```python
from build123d import *

# Parameters (mm, degrees)
EXTRUDE_1_DEPTH = 30


with BuildPart() as part:
    # 草图1 → 凸台-拉伸1 (new body)
    with BuildSketch(Plane.XY):
        with BuildLine():
            Line((-89.550424061, 9.743331503), (-65.958441791, 33.335313773))
            Line((-65.958441791, 33.335313773), (14.763144604, -47.386272621))
            add(Edge.make_bspline(
                [(14.763144604, -47.386272621), (0.494407811, -57.892318184), (-24.857012127, -59.689840271), (-58.186688521, -56.851240275), (-88.692238529, -45.382338902), (-109.075510722, -32.199451169), (-119.928178624, -20.63442306)],
                knots=[0, 0, 0, 0, 0.341115549, 0.507979438, 0.680177262, 1, 1, 1, 1], degree=3))
            Line((-119.928178624, -20.63442306), (-140.199044416, -40.51331885))
            add(Edge.make_bspline(
                [(-140.199044416, -40.51331885), (-132.851023827, -52.488780749), (-122.952075778, -62.464006208)],
                knots=[0, 0, 0, 1, 1, 1], degree=2))
            Line((-122.952075778, -62.464006208), (-124.511456774, -64.591840844))
            ThreePointArc((-124.511456774, -64.591840844), (-142.61936624, -98.390264744), (-108.909761073, -80.117542921))
            Line((-108.909761073, -80.117542921), (-106.018688387, -77.202324863))
            add(Edge.make_bspline(
                [(-106.018688387, -77.202324863), (-93.714859758, -86.031565942), (-72.92911338, -97.233004689), (-42.077489767, -104.91243417), (-17.024761238, -104.223351741), (14.056661387, -100.072035401), (36.008728716, -91.143735824), (47.83817857, -82.224550687)],
                knots=[0, 0, 0, 0, 0.276360348, 0.427878613, 0.575006209, 0.731440466, 1, 1, 1, 1], degree=3))
            Line((47.83817857, -82.224550687), (69.622057976, -103.828004523))
            Line((69.622057976, -103.828004523), (103.685759612, -69.479813065))
            Line((103.685759612, -69.479813065), (81.901880206, -47.876359228))
            add(Edge.make_bspline(
                [(-25.095901705, 146.484591642), (-10.567098374, 145.498050051), (11.160613299, 144.072831183), (37.531334045, 132.583388034), (55.897612016, 123.332823339), (71.537157173, 108.672601965), (84.710460364, 92.54260553), (97.252459301, 72.155728995), (105.276260592, 44.815754295), (107.60340097, 1.722304289), (97.111827436, -31.457580928), (81.901880206, -47.876359228)],
                knots=[0, 0, 0, 0, 0.159868672, 0.229200296, 0.310741288, 0.380982582, 0.45929677, 0.536185558, 0.638541511, 0.764116301, 1, 1, 1, 1], degree=3))
            add(Edge.make_bspline(
                [(-25.095901705, 146.484591642), (-8.963236942, 140.754746766), (13.87303757, 127.036506772), (36.100717553, 101.745358423), (48.669739491, 80.953224615), (56.825285706, 59.482294206), (60.519405197, 37.995942764), (60.521784194, 11.949353151), (56.293651863, -6.693592279), (47.83817857, -16.161590205)],
                knots=[0, 0, 0, 0, 0.253918506, 0.386919221, 0.496446637, 0.613180361, 0.7259311, 0.817885326, 1, 1, 1, 1], degree=3))
            Line((47.83817857, -16.161590205), (-33.345995712, 65.022584077))
            Line((-33.345995712, 65.022584077), (-2.121313296, 96.247266493))
            Line((-2.121313296, 96.247266493), (-22.475180352, 116.60113355))
            ThreePointArc((-22.475180352, 116.60113355), (-41.533061284, 110.257723938), (-61.563856858, 111.74396073))
            Line((-61.563856858, 111.74396073), (-126.557455073, 46.750362515))
            Line((-126.557455073, 46.750362515), (-89.550424061, 9.743331503))
        make_face()
    extrude(amount=EXTRUDE_1_DEPTH)


solid = part.part
```
CAD build for the part. Positions are in the model's coordinates, mm. A direction names the side the tool comes from. Round coordinates to 2 decimals unless told otherwise and drop trailing zeros.
Q1. Slice it at A-A (x = 11). State how many separate pieces and enclosed holes the cut face has, and give its area (3 significant figures).
Q2. Which spindle directions (+Z, -Z, +X, -X, +Y, -Y) get a long thin tool onto all of the face, cutting with end or side? Do faces 5 (the flat face through (6, -5, 0)), 6 (the flat face through (7.814, 23.862, 14.79)), 7 (the flat face through (-129.922, -30.435, 14.79)), 8 (the flat face through (58.6, -92.9, 14.8)). Say none if no direction does.
Q3. Drop flat-ended pins along their axis: pin 1 (4 mm diameter, centred on y = -2, z = 20.5, fed in from -X); pin 2 (4 mm diameter, centred on x = -48.5, z = 6, fed in from +Y); pin 3 (10 mm diameter, centred on x = -59, z = 4, fed in from +Y). Give the stop position or say it passes through.
Q4. Wall check: L1, parallel to X at y = 18.5, z = 9.5; L2, parallel to X at y = 19, z = 14; L3, parallel to X at y = 5, z = 21. Give the ranges that are in metal, low to high.
Q5. Two-plate mould, pull along X, no slides. Class faces 1 (the flat face through (92.946, -58.829, 14.79)), 2 (the flat face through (-26.163, -6.46, 14.79)), 3 (the flat face through (-93.61, 79.7, 14.79)), 4 (the flat face through (6, -5, 30)): pulls with the +X half, pulls with the -X half, needs draft (parallel to the pull), parting line crosses it, or undercut.
Results below:
1. separate pieces: 3
1. enclosed holes: 0
1. area: 3,880 mm2
2. face 5: -Z, +X, -X, +Y, -Y
2. face 6: +Z, -Z
2. face 7: +Z, -Z, -X
2. face 8: +Z, -Z, -Y
3. pin 1: stops at x = -32.62
3. pin 2: stops at y = 109.94
3. pin 3: stops at y = 111.74
4. L1: x = -98.31 to -80.79, -51.12 to 13.18, 60.08 to 105.89
4. L2: x = -98.81 to -80.29, -51.62 to 12.68, 60.12 to 105.9
4. L3: x = -37.62 to 26.68, 58.17 to 104.86
5. face 1: pulls with the +X half
5. face 2: undercut
5. face 3: pulls with the -X half
5. face 4: needs draft
